Source: CAD feature listing. Evaluate the final solid. Frame: model axes, mm. A direction names the side the tool comes from. Round coordinates to 2 decimals unless told otherwise and drop trailing zeros. Loops run counter-clockwise (first coordinate to the right, second up) from the corner with the lowest first, then second, coordinate; pieces in that order, holes last. Notation, with made-up numbers: M 74,-37.5 L 107,-37.5 A32 ccw 107,-1.5 Z; hole C -1.5,76 d1. An arc over 180 degrees is marked long. Write each question's results on one line, items separated by ' | '. Start each with the question number.
1. Section B-B on z = 1.5. Output: boundary loops of the cut face in (x, y), and give its area (3 significant figures).
2. Section A-A on x = -46. Output: boundary loops of the cut face in (y, z).
3. Section D-D on x = -11.5. Output: boundary loops of the cut face in (y, z).
4. Section C-C on y = 3.25. Give the number of separate pieces and of enclosed holes in the cut face, and give its area (3 significant figures).
5. Ray query, line 1 (X direction, y = 5.5, z = 0); line 2 (X direction, y = 7.25, z = -14); line 3 (X direction, y = 8.25, z = -38.5). Return the intervals inside material, ascending.
6. Contact query for flat-ended pins moving along their axis: pin 1 Ø8.5 at (y, z) = (4.5, -57) entering from +X; pin 2 Ø6 at (x, y) = (15.5, 13) entering from -Z; pin 3 Ø5 at (x, z) = (-11.5, -54) entering from -Y; pin 4 Ø6 at (x, y) = (17.5, 11) entering from -Z. Output: stop coordinate, or through.
7. Set-up query: faces 1 (the flat face through (-13, 9, -57)), 2 (the cylindrical face through (-9.106, 8.507, -59.773)), 3 (the flat face through (-26.5, 4, -51)). Return all of +Z, -Z, +X, -X, +Y, -Y with unobstructed straight access to the full face (end or side cutting, diameter ignored); none if empty.
8. Draft query along Z for faces 4 (the flat face through (-4, 0, -13)), 5 (the cylindrical face through (17.07, 7.89, -0.65)), 6 (the cylindrical face through (9.41, 8.112, 11.004)), 7 (the cylindrical face through (-13.034, 15.825, -28.36)). Return one class per face: released by +Z, released by -Z, zero draft, split by the parting line, or undercut.
from build123d import *

# Parameters (mm, degrees)
SKETCH_1_R          = 3
EXTRUDE_1_DEPTH     = 16
SKETCH_5_W          = 20
SKETCH_5_H          = 8
REVOLVE_1_ANGLE     = 180
SKETCH_6_R          = 3
CUT_EXTRUDE_4_DEPTH = 20
CUT_EXTRUDE_3_DEPTH = 30
SKETCH_7_R          = 3
CUT_EXTRUDE_5_DEPTH = 85.118812266
EXTRUDE_START       = 1
SKETCH_9_R          = 6.25
SKETCH_9_R_2        = 3
EXTRUDE_2_DEPTH     = 1
FILLET_1_R          = 10
FILLET_START        = -52
FILLET_2_DEPTH      = 79
FILLET_START_2      = -26.5
FILLET_2_2_DEPTH    = 30


with BuildPart() as part:
    # 草图1 → 凸台-拉伸1 (new body)
    with BuildSketch(Plane(origin=(0, 0, 0), x_dir=(1, 0, 0), z_dir=(0, 1, 0))):
        Polygon((-54, -10.000198617), (-29, -10.000198617), (-21.5, -23), (-21.5, -40), (-1.5, -40), (-1.5, -23), (9, -10.000198617), (29, -10.000198617), (29, 28.999801383), (3.5, 28.999801383), (3.5, 63.999801383), (-26.5, 63.999801383), (-26.5, 28.999801383), (-54, 28.999801383), align=None)
        with Locations(Location((-46, 14, 0), (0, 0, 270))):
            Circle(SKETCH_1_R, mode=Mode.SUBTRACT)
        with Locations(Location((20, 0, 0), (0, 0, 270))):
            Circle(SKETCH_1_R, mode=Mode.SUBTRACT)
        with BuildLine():
            Line((-30.266898407, 6.075760101), (-4.266898407, -7.924239899))
            ThreePointArc((-4.266898407, -7.924239899), (7.924239899, -4.266898407), (4.266898407, 7.924239899))
            Line((4.266898407, 7.924239899), (-21.733101593, 21.924239899))
            ThreePointArc((-21.733101593, 21.924239899), (-33.924239899, 18.266898407), (-30.266898407, 6.075760101))
        make_face(mode=Mode.SUBTRACT)
    extrude(amount=EXTRUDE_1_DEPTH)

    # 草图5 → 旋转1 (revolve)
    with BuildSketch(Plane.XY.offset(40)):
        with Locations((-11.5, 12)):
            Rectangle(SKETCH_5_W, SKETCH_5_H)
    revolve(axis=Axis((-21.5, 8, 40), (1, 0, 0)), revolution_arc=REVOLVE_1_ANGLE)

    # 草图6 → 切除-拉伸4 (cut)
    with BuildSketch(Plane(origin=(-1.5, 0, 0), x_dir=(0, 0, -1), z_dir=(1, 0, 0))):
        with Locations((-40, 8)):
            Circle(SKETCH_6_R)
    extrude(amount=-CUT_EXTRUDE_4_DEPTH, mode=Mode.SUBTRACT)

    # 草图4 → 切除-拉伸3 (cut)
    with BuildSketch(Plane(origin=(3.5, 0, 0), x_dir=(0, 0, -1), z_dir=(1, 0, 0))):
        Polygon((28.999801383, 16), (63.999801383, 16), (63.999801383, 8), (43.999801383, 8), align=None)
    extrude(amount=-CUT_EXTRUDE_3_DEPTH, mode=Mode.SUBTRACT)

    # 草图7 → 切除-拉伸5 (cut, through all)
    with BuildSketch(Plane(origin=(0, 8, 0), x_dir=(1, 0, 0), z_dir=(0, 1, 0))):
        with Locations(Location((-11.5, 53.999801383, 0), (0, 0, 270))):
            Circle(SKETCH_7_R)
    extrude(amount=-CUT_EXTRUDE_5_DEPTH, mode=Mode.SUBTRACT)

    # 草图9 → 凸台-拉伸2 (add)
    with BuildSketch(Plane(origin=(0, 8, 0), x_dir=(1, 0, 0), z_dir=(0, 1, 0)).offset(EXTRUDE_START)):
        with Locations(Location((-11.5, 53.999801383, 0), (0, 0, 90))):
            Circle(SKETCH_9_R)
        with Locations(Location((-11.5, 53.999801383, 0), (0, 0, 270))):
            Circle(SKETCH_9_R_2, mode=Mode.SUBTRACT)
    extrude(amount=-EXTRUDE_2_DEPTH)

    # 圆角1
    fillet_1_edges = [part.edges().sort_by_distance(p)[0] for p in [
        (-21.5, 8, 23),
        (-29, 8, 10.000198617),
        (-54, 8, 10.000198617),
        (-54, 8, -28.999801383),
        (-26.5, 8, -28.999801383),
        (3.5, 8, -28.999801383),
        (29, 8, -28.999801383),
        (29, 8, 10.000198617),
        (9, 8, 10.000198617),
        (-1.5, 8, 23),
    ]]
    fillet(fillet_1_edges, radius=FILLET_1_R)

    # 圆角2: read off the stored shape, not the designer's step
    # 圆角2 outline → 圆角2 (cut)
    with BuildSketch(Plane.YZ.offset(FILLET_START)):
        with BuildLine():
            Line((14.823529412, -31.205683736), (16, -28.999801383))
            Line((16, -28.999801383), (16, -26.499801383))
            ThreePointArc((16, -26.499801383), (15.701425001, -28.925157633), (14.823529412, -31.205683736))
        make_face()
    extrude(amount=FILLET_2_DEPTH, mode=Mode.SUBTRACT)

    # Fillet 2 2 outline → Fillet 2 2 (add)
    with BuildSketch(Plane.YZ.offset(FILLET_START_2)):
        with BuildLine():
            Line((8, -43.999801383), (8, -46.499801383))
            ThreePointArc((8, -46.499801383), (8.298574999, -44.074445133), (9.176470588, -41.79391903))
            Line((9.176470588, -41.79391903), (8, -43.999801383))
        make_face()
    extrude(amount=FILLET_2_2_DEPTH)


solid = part.part
Taken from the geometry:
1) outline: M -53.89,0 L -16.2,0 L -16.2,16 L -53.89,16 Z; M 8.87,0 L 17.4,0 L 17.4,16 L 8.87,16 Z; M 22.6,0 L 28.89,0 L 28.89,16 L 22.6,16 Z | area: 840 mm^2
2) outline: M 0,-28.8 L 15.73,-28.8 A10 ccw 16,-26.5 L 16,-17 L 0,-17 Z; M 0,-11 L 16,-11 L 16,9.8 L 0,9.8 Z
3) outline: M 0,-64 L 8,-64 L 8,-60.25 L 9,-60.25 L 9,-57 L 0,-57 Z; M 0,-51 L 9,-51 L 9,-47.75 L 8,-47.75 L 8,-46.5 A10 cw 9.18,-41.79 L 14.82,-31.21 A10 ccw 16,-26.5 L 16,-16.41 L 0,-16.41 Z; M 0,4.03 L 16,4.03 L 16,40 A8 ccw 0,40 Z; hole C 8,40 d6
4) separate pieces: 1 | enclosed holes: 4 | area: 4,230 mm^2
5) line 1: -54 to -18.98, 9 to 17, 23 to 29 | line 2: -54 to -49, -43 to -35, -7.02 to 29 | line 3: -26.51 to 3.51
6) pin 1: x = 3.5 | pin 2: z = -29.05 | pin 3: through | pin 4: z = -29
7) face 1: -Z, +X, -X, +Y | face 2: +Y | face 3: -Z, -X, +Y, -Y
8) face 4: zero draft | face 5: undercut | face 6: released by +Z | face 7: released by -Z
